Autodesk Inventor part; units mm, degrees
ref_plane "YZ Plane" through (0, 0, 0) normal (1, 0, 0) x (0, 1, 0)
ref_plane "XZ Plane" through (0, 0, 0) normal (0, 1, 0) x (-1, 0, 0)
ref_plane "XY Plane" through (0, 0, 0) normal (0, 0, 1) x (1, 0, 0)
sketch "Sketch1" plane through (0, 0, 0) normal (0, 0, 1) x (1, 0, 0)
  circle A0 centre (0, 0) radius 3.6957
  dimension "d0" = 7.3914
extrude "Extrusion1" add sketch "Sketch1" along normal blind 4.0386
sketch "Sketch2" plane through (0, 0, 4.0386) normal (0, 0, 1) x (1, 0, 0)
  circle A0 centre (0, 0) radius 3.6957
  circle A1 centre (0, 0) radius 2.4003
  dimension "d3" = 1.2954
extrude "Extrusion2" cut sketch "Sketch2" against normal blind 2.7432 contours A1
sketch "Sketch3" plane through (0, 0, 0) normal (0, 0, -1) x (-1, 0, 0)
  circle A0 centre (0, 0) radius 3.6957
  circle A1 centre (0, 0) radius 2.1717
  dimension "d6" = 1.524
extrude "Extrusion3" cut sketch "Sketch3" against normal blind 1.0668 contours A1
sketch "Sketch4" plane through (0, 0, 1.2954) normal (0, 0, 1) x (1, 0, 0)
  circle A0 centre (0, 0) radius 2.4003
  circle A1 centre (0, 0) radius 1.4478
  dimension "d9" = 2.8956
extrude "Extrusion4" cut sketch "Sketch4" against normal through all contours A1
ref_plane "Work Plane1" through (0, 0, 0.5334) normal (0, 0, -1) x (-1, 0, 0)
sketch "Sketch5" plane through (0, 0, 0.5334) normal (0, 0, -1) x (-1, 0, 0)
  circle A0 centre (0, 0) radius 3.6957
  line L0 (-2.3894, 2.8194) -> (-14.0061, 2.032)
  line L1 (-2.3894, -2.8194) -> (-14.0061, -2.032)
  arc A1 (-14.0061, 2.032) -> (-14.0061, -2.032) centre (-13.8684, 0) ccw
  circle A2 centre (0, 0) radius 2.4003
  line L2 (2.3894, 2.8194) -> (14.0061, 2.032)
  arc A3 (14.0061, -2.032) -> (14.0061, 2.032) centre (13.8684, 0) ccw
  line L3 (2.3894, -2.8194) -> (14.0061, -2.032)
  dimension "d12" = 5.6388
  dimension "d13" = 4.064
  dimension "d15" = 13.8684
  dimension "d28" = 360
extrude "Extrusion5" add sketch "Sketch5" along normal mid plane 1.0668 contours A0 L1 A1 L0
sketch "Sketch6" plane through (0, 0, 0) normal (0, 0, -1) x (-1, 0, 0)
  circle A0 centre (0, 0) radius 2.1717
  circle A1 centre (-15.1836, 0) radius 0.2611
  circle A2 centre (-12.9992, 0) radius 0.2611
  circle A3 centre (-10.8148, 0) radius 0.2611
  circle A4 centre (-8.6304, 0) radius 0.2611
  circle A5 centre (-6.446, 0) radius 0.2611
  circle A6 centre (-4.2616, 0) radius 0.2611
  dimension "d18" = 1.8288
  dimension "d19" = 4.0132
  dimension "d20" = 2.1844
  dimension "d21" = 2.1844
  dimension "d22" = 2.1844
  dimension "d23" = 2.1844
extrude "Extrusion6" cut sketch "Sketch6" against normal through all contours A1 | A2 | A3 | A4 | A5 | A6
pattern_circular "Circular Pattern1" count 2 over 360 about axis through (0, 0, 0) along (0, 0, 1) of "Extrusion5", "Extrusion6"
properties part number "Servo Horn"
Verification items for the finished model (mm, model axes). A direction names the side the tool comes from. Coordinates: 2 decimals unless noted, no trailing zeros. Loops run counter-clockwise (first coordinate to the right, second up) from the corner with the lowest first, then second, coordinate; pieces in that order, holes last. Notation, with made-up numbers: M 67,60.25 L 123,60.25 A25 ccw 123,74.25 Z; hole C 56,-20.5 d3. An arc over 180 degrees is marked long. One line per item, written item: value.
1. Mould release check, pull along Y, two halves, no side actions. Record for faces 3 (the flat face through (8.12, -2.43, 0.54)), 4 (the cylindrical face through (15.905, -0.043, 0.541)), 5 (the cylindrical face through (-0.31, 2.38, 2.69)), 6 (the cylindrical face through (0.47, -2.12, 0.53)): pulls with the +Y half, pulls with the -Y half, needs draft (parallel to the pull), parting line crosses it, or undercut.
Answers follow:
face 3: pulls with the -Y half
face 4: parting line crosses it
face 5: undercut
face 6: undercut
2. Gauge pin test, flat ends, axial feed: P1, Ø2.5, axis at x = 0, y = 0, coming from the -Z side; P2, Ø4, axis at x = -5, y = -1, coming from the +Z side; P3, Ø1.7, axis at x = 12.5, y = -0.5, coming from the +Z side; P4, Ø1.4, axis at x = 0, y = -1, coming from the +Z side. Record the tip position at first contact, or that the pin passes through.
Answers follow:
P1: through
P2: z = 4.04
P3: z = 1.07
P4: z = 1.3
3. Section check B-B on z = 2.3. Record the cut outline in (x, y), plus the area to 3 significant figures.
Answers follow:
outline: C 0,0 d7.39; hole C 0,0 d4.8
area: 24.8 mm^2
4. Section check D-D on x = 12. Record the cut outline in (y, z), plus the area to 3 significant figures.
Answers follow:
outline: M -2.17,0 L 2.17,0 L 2.17,1.07 L -2.17,1.07 Z
area: 4.63 mm^2
5. Material ranges on line 1 along Y through (x, z) = (0, 2.55); line 2 along Z through (x, y) = (-12, -0.5); line 3 along Y through (x, z) = (1, 1.4), recorded low to high. Write a range as from..to.
Answers follow:
line 1: -3.7..-2.4, 2.4..3.7
line 2: 0..1.07
line 3: -3.56..-2.18, 2.18..3.56
6. Section check A-A on x = 0. Record the cut outline in (y, z).
Answers follow:
outline: M -3.7,0 L -2.17,0 L -2.17,1.07 L -1.45,1.07 L -1.45,1.3 L -2.4,1.3 L -2.4,4.04 L -3.7,4.04 Z; M 1.45,1.07 L 2.17,1.07 L 2.17,0 L 3.7,0 L 3.7,4.04 L 2.4,4.04 L 2.4,1.3 L 1.45,1.3 Z
7. Set-up check for faces 1 (the flat face through (0, -2, 1.295)), 2 (the flat face through (-8.12, -2.43, 0.54)): record each of +Z, -Z, +X, -X, +Y, -Y from which the full face is reachable in a straight line by a thin tool's end or side.
Answers follow:
face 1: +Z
face 2: +Z, -Z, -X, -Y
8. Section check C-C on y = 1.75. Record the cut outline in (x, z).
Answers follow:
outline: M -14.91,0 L -1.29,0 L -1.29,1.07 L 1.29,1.07 L 1.29,0 L 14.91,0 L 14.91,1.07 L 3.26,1.07 L 3.26,4.04 L 1.64,4.04 L 1.64,1.3 L -1.64,1.3 L -1.64,4.04 L -3.26,4.04 L -3.26,1.07 L -14.91,1.07 Z
